Study the drawing (mm; zero at the part's minimum x, y, z) and answer. A direction names the side the tool comes from. Coordinates: 2 decimals unless noted, no trailing zeros. Order: outer loops, then holes, each group sorted by start corner. A loop starts at its lowest first (then second) coordinate and runs counter-clockwise, first axis right, second up. Notation, with made-up numbers: (30.25, 87) - (70.25, 87) arc R28 cw to (70.25, 121) - close; hole circle Ø10 at (62.5, 28). An arc over 180 degrees is marked (long way). Write item = value, one per line.
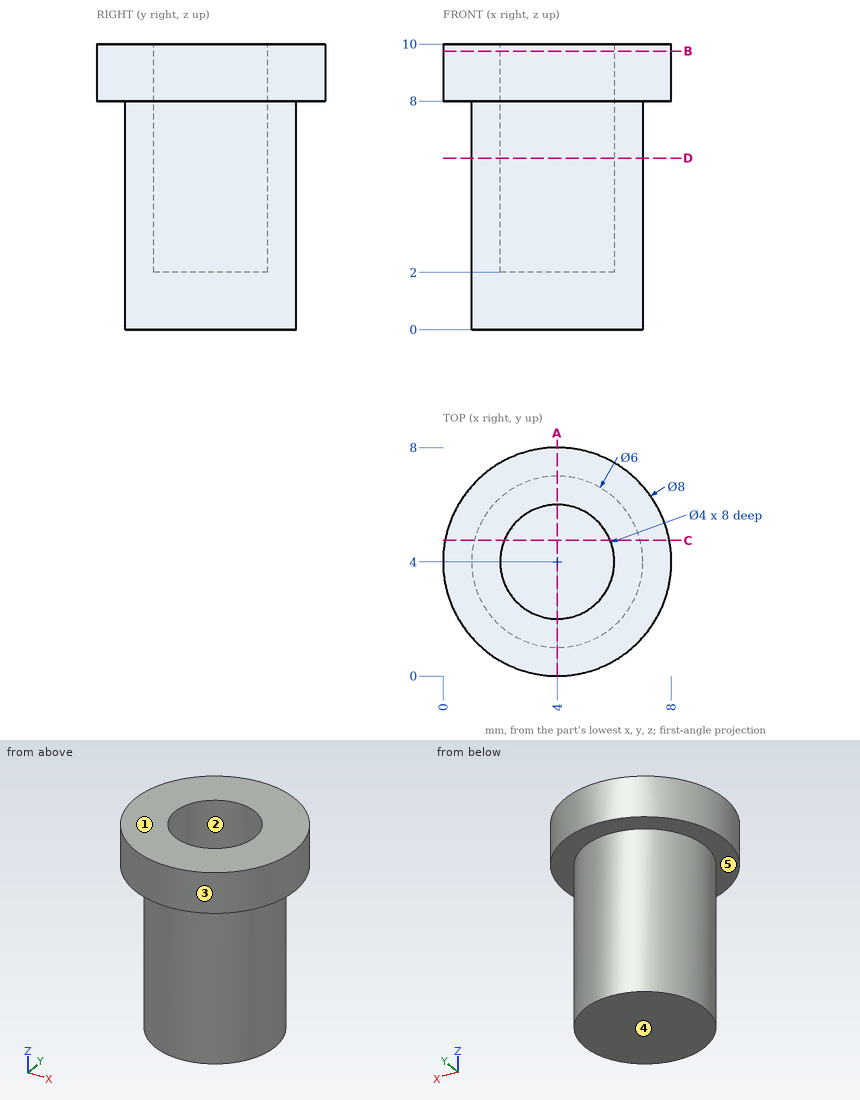
1) The part is cut by section D-D (z = 6). Determine the outline of the cut face in (x, y).
Returned:
outline = circle Ø6 at (4, 4); hole circle Ø4 at (4, 4)
2) Flat-ended cylindrical pins translate along their axes: pin 1 Ø2 at (x, z) = (2.5, 8) entering from -Y; pin 2 Ø3.5 at (x, y) = (4, 4) entering from -Z; pin 3 Ø4 at (x, z) = (5.5, 1.5) entering from -Y; pin 4 Ø2 at (x, z) = (6, 7.5) entering from +Y. Find the tip coordinate at first contact, or state that the pin passes through.
Returned:
pin_1 = 0.03
pin_2 = 0
pin_3 = 1
pin_4 = 7.84
3) The part is cut by section A-A (x = 4). Determine the outline of the cut face in (y, z).
Returned:
outline = (0, 8) - (1, 8) - (1, 0) - (7, 0) - (7, 8) - (8, 8) - (8, 10) - (6, 10) - (6, 2) - (2, 2) - (2, 10) - (0, 10) - close
4) For the marked faces 4 and 5, determine the directions among +Z, -Z, +X, -X, +Y, -Y from which every point of the face is accessible in a straight line to the end or side of a thin tool.
Returned:
face_4 = -Z, +X, -X, +Y, -Y
face_5 = -Z
5) Straight lines are drawn through the part: line 1 along Y through (x, z) = (4, 6); line 2 along Y through (x, z) = (4, 9.5); line 3 along Z through (x, y) = (4.5, 4). For each, find the intervals that lie inside material, in ascending order. Write a range as from..to.
Returned:
line_1 = 1..2, 6..7
line_2 = 0..2, 6..8
line_3 = 0..2
6) The part is cut by section B-B (z = 9.75). Determine the outline of the cut face in (x, y).
Returned:
outline = circle Ø8 at (4, 4); hole circle Ø4 at (4, 4)
7) The part is cut by section C-C (y = 4.75). Determine the outline of the cut face in (x, z).
Returned:
outline = (0.07, 8) - (1.1, 8) - (1.1, 0) - (6.9, 0) - (6.9, 8) - (7.93, 8) - (7.93, 10) - (5.85, 10) - (5.85, 2) - (2.15, 2) - (2.15, 10) - (0.07, 10) - close
8) Determine the mould class of the marked faces 1, 2 and 3 for opening direction X: pulls with the +X half, pulls with the -X half, needs draft (parallel to the pull), parting line crosses it, or undercut.
Returned:
face_1 = needs draft
face_2 = undercut
face_3 = parting line crosses it
